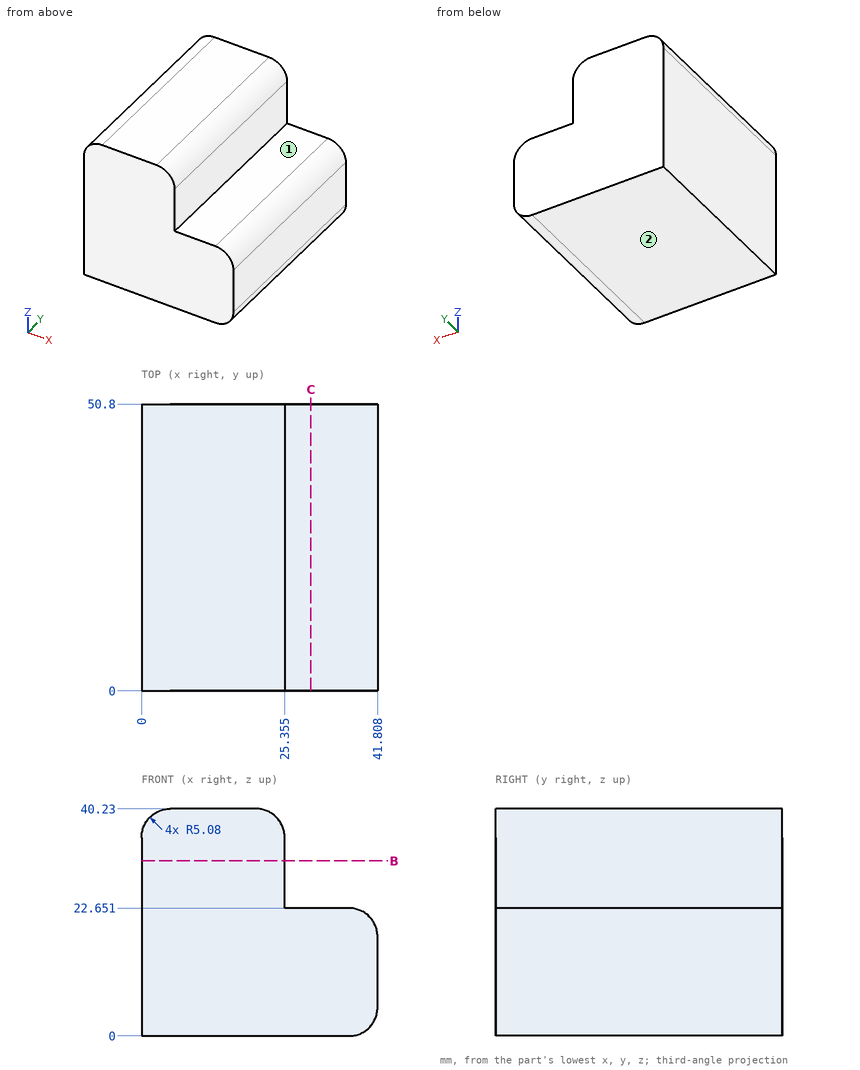
Check sheet for the drawn part. Datum: minimum x, y, z corner. Units: mm. A direction names the side the tool comes from. Coordinates: 2 decimals unless noted, no trailing zeros. Order: outer loops, then holes, each group sorted by start corner. A loop starts at its lowest first (then second) coordinate and runs counter-clockwise, first axis right, second up. Notation, with made-up numbers: (25, 41) -> (58, 41) arc R15 ccw to (58, 56) -> close; hole circle Ø5 at (49.5, -39). An arc over 180 degrees is marked (long way). Use a Markdown table: item, result. Add a question column.
1. Cross-section at B-B (z = 31). Enter the section's corners in (x, y) (1 decimal), and give its area (3 significant figures).
2. Cross-section at C-C (x = 30). Enter the section's corners in (y, z).
3. Go/stop test with flat-tipped pins: pin 1 Ø9 at (x, y) = (31.5, 15) entering from +Z; pin 2 Ø8 at (y, z) = (39.5, 25) entering from +X (1 decimal); pin 3 Ø4 at (y, z) = (20, 33) entering from +X (1 decimal). Record where each tip stops, or that it passes through.
4. Material ranges on L1, parallel to Z at x = 29.5, y = 36.5; L2, parallel to X at y = 34.5, z = 30 (1 decimal); L3, parallel to X at y = 19.5, z = 5, recorded low to high.
5. Set-up check for the marked faces 1 and 2: record each of +Z, -Z, +X, -X, +Y, -Y from which the full face is reachable in a straight line by a thin tool's end or side.
Filled sheet:
| question | item | result |
|---|---|---|
| 1 | outline | (0, 0) -> (25.4, 0) -> (25.4, 50.8) -> (0, 50.8) -> close |
| 1 | area | 1,290 mm2 |
| 2 | outline | (0, 0) -> (50.8, 0) -> (50.8, 22.65) -> (0, 22.65) -> close |
| 3 | pin 1 | z = 22.65 |
| 3 | pin 2 | x = 40.5 |
| 3 | pin 3 | x = 25.4 |
| 4 | L1 | 0 to 22.65 |
| 4 | L2 | 0 to 25.4 |
| 4 | L3 | 0 to 41.81 |
| 5 | face 1 | +Z, +X, +Y, -Y |
| 5 | face 2 | -Z, +X, -X, +Y, -Y |
